Can you work these out from the drawing? Everything is in mm from the part's minimum corner. Coordinates: 2 decimals unless noted, no trailing zeros. Write each loop counter-clockwise with the first axis right and the second up, starting at its lowest first coordinate (ties: lowest second). Pieces come first, ordered by that corner, then holes. Notation, with made-up numbers: (52.5, -29.75) -> (86.5, -29.75) arc R10 ccw to (86.5, -20.75) -> close; hole circle Ø6 at (-10, 60). An arc over 180 degrees is marked (long way). Use CSV: the item, a comma, the result in double quotes. Start each with the question number.
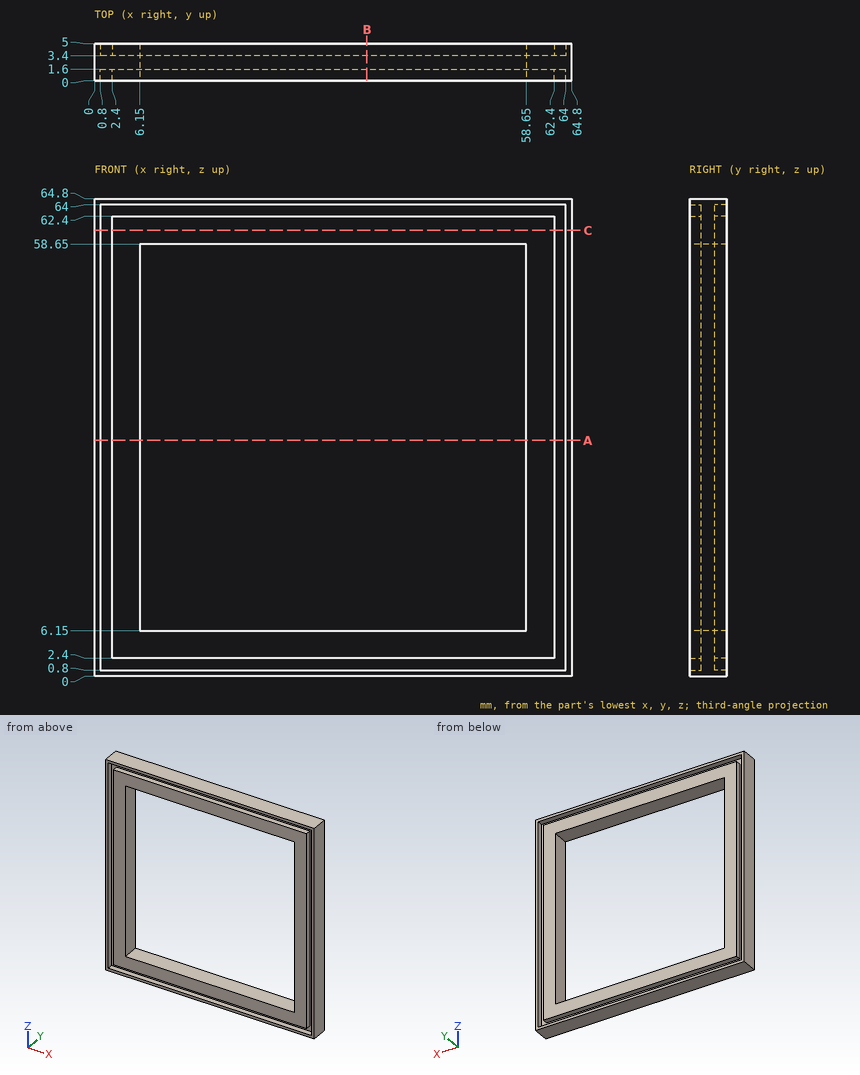
Item 1: If I drill on line 1 along Z through (x, y) = (52.5, 1.2); line 2 along Z through (x, y) = (62.5, 4.8), over which ranges is the centre line in solid material (lowest first)?
Item 2: I want a section at A-A on z = 32. Please give me the cut outline in (x, y).
Item 3: I'm going to push a flat-ended pin straight in: pin 1 (12 mm diameter, centred on x = 15, z = 19, fed in from -Y). Where does the tip first touch, or does it pass through?
Item 4: I want a section at B-B on x = 37. Please give me the cut outline in (y, z), then the cut area to 3 significant figures.
Item 5: I want a section at C-C on z = 60.5. Please give me the cut outline in (x, y).
Geometry says:
1,line 1,"0 to 0.8, 2.4 to 6.15, 58.65 to 62.4, 64 to 64.8"
1,line 2,"0 to 0.8, 64 to 64.8"
2,outline,"(0, 0) -> (0.8, 0) -> (0.8, 1.6) -> (2.4, 1.6) -> (2.4, 0) -> (6.15, 0) -> (6.15, 5) -> (2.4, 5) -> (2.4, 3.4) -> (0.8, 3.4) -> (0.8, 5) -> (0, 5) -> close; (58.65, 0) -> (62.4, 0) -> (62.4, 1.6) -> (64, 1.6) -> (64, 0) -> (64.8, 0) -> (64.8, 5) -> (64, 5) -> (64, 3.4) -> (62.4, 3.4) -> (62.4, 5) -> (58.65, 5) -> close"
3,pin 1,"through"
4,outline,"(0, 0) -> (5, 0) -> (5, 0.8) -> (3.4, 0.8) -> (3.4, 2.4) -> (5, 2.4) -> (5, 6.15) -> (0, 6.15) -> (0, 2.4) -> (1.6, 2.4) -> (1.6, 0.8) -> (0, 0.8) -> close; (0, 58.65) -> (5, 58.65) -> (5, 62.4) -> (3.4, 62.4) -> (3.4, 64) -> (5, 64) -> (5, 64.8) -> (0, 64.8) -> (0, 64) -> (1.6, 64) -> (1.6, 62.4) -> (0, 62.4) -> close"
4,area,"51.3 mm2"
5,outline,"(0, 0) -> (0.8, 0) -> (0.8, 1.6) -> (2.4, 1.6) -> (2.4, 0) -> (62.4, 0) -> (62.4, 1.6) -> (64, 1.6) -> (64, 0) -> (64.8, 0) -> (64.8, 5) -> (64, 5) -> (64, 3.4) -> (62.4, 3.4) -> (62.4, 5) -> (2.4, 5) -> (2.4, 3.4) -> (0.8, 3.4) -> (0.8, 5) -> (0, 5) -> close"
